Source: three-view drawing plus pictorial views. Frame: mm from the lowest corner of the part. Give positions to 0.01 mm unless a question says otherwise; leave off trailing zeros. Write each loop counter-clockwise with the first axis right and the second up, starting at its lowest first coordinate (ties: lowest second). Pieces come first, ordered by that corner, then holes. Notation, with made-up numbers: (32.25, -28) - (62.25, -28) arc R26 cw to (62.25, -7) - close; hole circle Ø7 at (9.25, 43.25). An arc over 180 degrees is marked (long way). One line per question, with ' | ' between items. Start each with the question number.
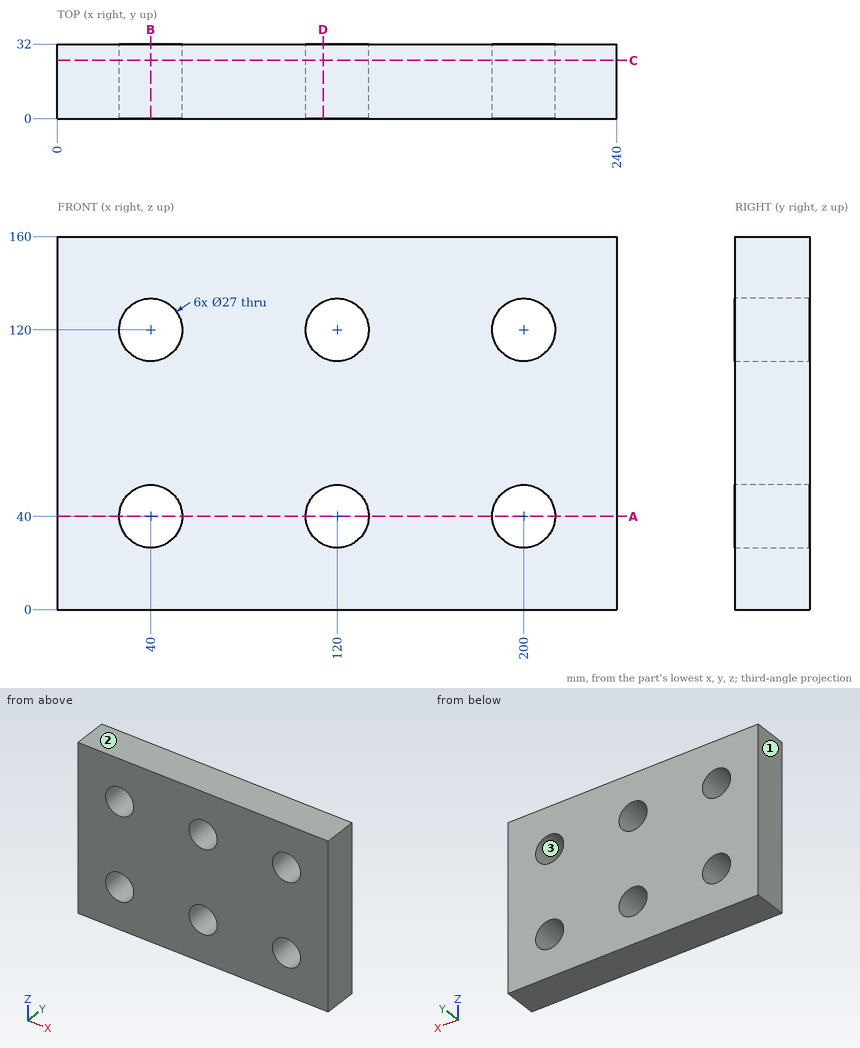
1) Line query: L1, parallel to X at y = 15, z = 120; L2, parallel to X at y = 22.5, z = 122.5; L3, parallel to Z at x = 46, y = 18. Output: solid intervals per line, ascending.
2) First-contact query: pin 1 Ø16 at (x, z) = (120, 120) entering from +Y. Flat tip, straight axial feed; report the tip coordinate or a pass-through.
3) Pull-direction query (Z, two-part tool) for the marked faces 1, 2 and 3; classes: +Z half, -Z half, draft (parallel to the pull), parting line (faces both ways), or undercut.
4) Section C-C, the plane y = 25. Output: boundary loops of the cut face in (x, z).
5) Section D-D, the plane x = 114. Output: boundary loops of the cut face in (y, z).
6) Section A-A, the plane z = 40. Output: boundary loops of the cut face in (x, y), plus the area to 3 significant figures.
7) Section B-B, the plane x = 40. Output: boundary loops of the cut face in (y, z).
Answer key:
1) L1: 0 to 26.5, 53.5 to 106.5, 133.5 to 186.5, 213.5 to 240 | L2: 0 to 26.73, 53.27 to 106.73, 133.27 to 186.73, 213.27 to 240 | L3: 0 to 27.91, 52.09 to 107.91, 132.09 to 160
2) pin 1: through
3) face 1: draft | face 2: +Z half | face 3: undercut
4) outline: (0, 0) - (240, 0) - (240, 160) - (0, 160) - close; hole circle Ø27 at (40, 40); hole circle Ø27 at (40, 120); hole circle Ø27 at (120, 40); hole circle Ø27 at (120, 120); hole circle Ø27 at (200, 40); hole circle Ø27 at (200, 120)
5) outline: (0, 0) - (32, 0) - (32, 27.91) - (0, 27.91) - close; (0, 52.09) - (32, 52.09) - (32, 107.91) - (0, 107.91) - close; (0, 132.09) - (32, 132.09) - (32, 160) - (0, 160) - close
6) outline: (0, 0) - (26.5, 0) - (26.5, 32) - (0, 32) - close; (53.5, 0) - (106.5, 0) - (106.5, 32) - (53.5, 32) - close; (133.5, 0) - (186.5, 0) - (186.5, 32) - (133.5, 32) - close; (213.5, 0) - (240, 0) - (240, 32) - (213.5, 32) - close | area: 5,090 mm^2
7) outline: (0, 0) - (32, 0) - (32, 26.5) - (0, 26.5) - close; (0, 53.5) - (32, 53.5) - (32, 106.5) - (0, 106.5) - close; (0, 133.5) - (32, 133.5) - (32, 160) - (0, 160) - close
